Design review of the part built by this model. Coordinates are the model's own, in mm. Face numbers are marked on the shaded views. A direction names the side the tool comes from. Coordinates: 2 decimals unless noted, no trailing zeros. Write each loop counter-clockwise with the first axis right and the second up, starting at its lowest first coordinate (ties: lowest second). Pieces come first, ordered by that corner, then holes. Notation, with made-up numbers: (68.25, 56.5) -> (79.25, 56.5) arc R23 ccw to (79.25, 66.5) -> close; hole circle Ø1 at (86, -21.75). An arc over 180 degrees is marked (long way). Write item = value, one per line. Start each with the question number.
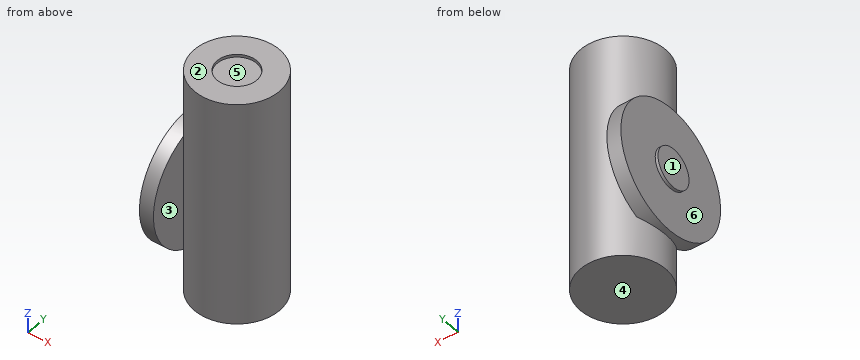
```python
from build123d import *

# Parameters (mm, degrees)
ESQUISSE1_R             = 150
BOSS_EXTRU_1_DEPTH      = 800
ESQUISSE2_R             = 225
BOSS_EXTRU_2_DEPTH      = 50
ESQUISSE4_R             = 70
ENL_V_MAT_EXTRU_2_DEPTH = 10
ESQUISSE3_R             = 70
BOSS_EXTRU_3_DEPTH      = 10


with BuildPart() as part:
    # Esquisse1 → Boss.-Extru.1 (new body)
    with BuildSketch(Plane.XY):
        Circle(ESQUISSE1_R)
    extrude(amount=-BOSS_EXTRU_1_DEPTH)

    # Esquisse2 → Boss.-Extru.2 (add)
    with BuildSketch(Plane(origin=(-120, 0, 0), x_dir=(0, 0, -1), z_dir=(1, 0, 0))):
        with Locations((450, 0)):
            Circle(ESQUISSE2_R)
    extrude(amount=-BOSS_EXTRU_2_DEPTH)

    # Esquisse4 → Enlèv. mat.-Extru.2 (cut)
    with BuildSketch(Plane.XY):
        Circle(ESQUISSE4_R)
    extrude(amount=-ENL_V_MAT_EXTRU_2_DEPTH, mode=Mode.SUBTRACT)

    # Esquisse3 → Boss.-Extru.3 (add)
    with BuildSketch(Plane.ZY.offset(170)):
        with Locations((-450, 0)):
            Circle(ESQUISSE3_R)
    extrude(amount=BOSS_EXTRU_3_DEPTH)


solid = part.part
```
(1) For the marked faces 4, 5 and 6, list the 3-axis set-ups (+Z, -Z, +X, -X, +Y, -Y) from which the entire face can be reached by the end or side of a thin tool; tool diameter is ignored.
(2) Take a section at D-D, the plane x = -36. State the section outline as (y, z) points, then the cut area to 3 significant figures.
(3) Take a section at B-B, the plane y = 0. State the section outline as (x, z) points, then the cut area to 3 significant figures.
(4) Take a section at C-C, the plane z = -450. State the section outline as (x, y) points, then the cut area to 3 significant figures.
(5) For line 1 (Y direction, x = 0, z = -5); line 2 (Z direction, x = -59.5, y = 13); line 3 (Y direction, x = 1, z = -477), list the stretches that pass through material, from the lowest coordinate up.
(6) Take a section at A-A, the plane x = 0. State the section outline as (y, z) points.
(7) For pin 1 Ø3 at (x, z) = (-77, -460) entering from +Y; pin 2 Ø10 at (y, z) = (130.5, -671.5) entering from +X; pin 3 Ø2 at (y, z) = (58, -146.5) entering from +X, all flat-tipped, find the tip position at first contact; note any pin that passes through.
(8) Mouldability with a two-part tool opening along X and no side actions: class the marked faces 1, 2 and 3 as pulls with the +X half, pulls with the -X half, needs draft (parallel to the pull), parting line crosses it, or undercut.
Report:
q1.face_4 = -Z, +X, -X, +Y, -Y
q1.face_5 = +Z
q1.face_6 = -X
q2.outline = (-145.62, -800) -> (145.62, -800) -> (145.62, 0) -> (60.03, 0) -> (60.03, -10) -> (-60.03, -10) -> (-60.03, 0) -> (-145.62, 0) -> close
q2.area = 232,000 mm2
q3.outline = (-180, -520) -> (-170, -520) -> (-170, -675) -> (-150, -675) -> (-150, -800) -> (150, -800) -> (150, 0) -> (70, 0) -> (70, -10) -> (-70, -10) -> (-70, 0) -> (-150, 0) -> (-150, -225) -> (-170, -225) -> (-170, -380) -> (-180, -380) -> close
q3.area = 249,000 mm2
q4.outline = (-180, -70) -> (-170, -70) -> (-170, -225) -> (-120, -225) -> (-120, -90) arc R150 ccw (long way) to (-120, 90) -> (-120, 225) -> (-170, 225) -> (-170, 70) -> (-180, 70) -> close
q4.area = 90,900 mm2
q5.line_1 = -150 to -70, 70 to 150
q5.line_2 = -800 to -10
q5.line_3 = -150 to 150
q6.outline = (-150, -800) -> (150, -800) -> (150, 0) -> (70, 0) -> (70, -10) -> (-70, -10) -> (-70, 0) -> (-150, 0) -> close
q7.pin_1 = 129.61
q7.pin_2 = 82.16
q7.pin_3 = 138.75
q8.face_1 = pulls with the -X half
q8.face_2 = needs draft
q8.face_3 = undercut
